Could you check a few things on this model? Use its own coordinates, in mm. A direction names the side the tool comes from. Round coordinates to 2 decimals unless told otherwise and drop trailing zeros. Write each loop counter-clockwise with the first axis right and the second up, starting at its lowest first coordinate (ties: lowest second). Pieces come first, ordered by that corner, then holes. Notation, with made-up numbers: (32, 3) -> (76, 3) arc R21 ccw to (76, 14) -> close; hole circle Ø11 at (-17.5, 71). An arc over 180 degrees is marked (long way). Return JSON: item names as keys, results as strings.
from build123d import *

# Parameters (mm, degrees)
F2_R            = 3.175
F3_DEPTH        = 22.226
F3_COPIES_COUNT = 6


# Not quite as in the source:
# - a pattern or mirror of a feature is missing from the dataset's text; its kind, count and spacing are read off the source's solid


with BuildPart() as f1:
    # F0 (on Front) → F1 (revolve)
    with BuildSketch(Plane.XZ):
        with BuildLine():
            Line((7.8105, 0), (34.1376, 0))
            Line((34.1376, 0), (34.1376, 22.225))
            Line((34.1376, 22.225), (16.6751, 22.225))
            Line((16.6751, 22.225), (16.6751, 14.224))
            ThreePointArc((16.6751, 14.224), (16.2287307345, 13.1463692655), (15.1511, 12.7))
            Line((15.1511, 12.7), (7.8105, 12.7))
            Line((7.8105, 12.7), (7.8105, 0))
        make_face()
    revolve(axis=Axis((0, 0, 6.35), (0, 0, 1)))

    # F2 (on face) → F3 (cut, through all)
    with BuildSketch(Plane.XY.offset(22.225)):
        with Locations((0, 26.2001)):
            Circle(F2_R)
    f3 = extrude(amount=-F3_DEPTH, mode=Mode.SUBTRACT)

    # F3_copies: F3 ×6 about axis
    f3_copies_axis = Axis((0, 0, 0), (0, 0, 1))
    for i in range(1, F3_COPIES_COUNT):
        add(f3.rotate(f3_copies_axis, i * 360 / F3_COPIES_COUNT), mode=Mode.SUBTRACT)


solid = f1.part
1) If I drill on probe 1 along Y at (x, z) = (0, 3); probe 2 along Y at (x, z) = (25.5, 13); probe 3 along X at (y, z) = (12.5, 8.5), over which ranges is the centre line in solid material (lowest first)? Write a range as [from, to].
Return value:
{"probe 1": "[-34.14, -29.38], [-23.03, -7.81], [7.81, 23.03], [29.38, 34.14]", "probe 2": "[-22.7, -14.58], [-11.62, 11.62], [14.58, 22.7]", "probe 3": "[-31.77, -25.81], [-19.57, 19.57], [25.81, 31.77]"}
2) Will these pins go through, and if not, where does the flat tip stop? pin 1 Ø4 at (x, y) = (22.69, 13.1) entering from -Z; pin 2 Ø10 at (x, y) = (0, 26.2) entering from +Z (3 decimals); pin 3 Ø3 at (x, z) = (2.5, 5) entering from -Y; pin 4 Ø8 at (y, z) = (16, 7.5) entering from -X.
Return value:
{"pin 1": "through", "pin 2": "z = 22.225", "pin 3": "y = -34.12", "pin 4": "x = -31.96"}
3) I want a section at A-A, the plane y = 0. Please give me the cut outline in (x, z) (1 decimal).
Return value:
{"outline": "(-34.1, 0) -> (-7.8, 0) -> (-7.8, 12.7) -> (-15.2, 12.7) arc R1.5 cw to (-16.7, 14.2) -> (-16.7, 22.2) -> (-34.1, 22.2) -> close; (7.8, 0) -> (34.1, 0) -> (34.1, 22.2) -> (16.7, 22.2) -> (16.7, 14.2) arc R1.5 cw to (15.2, 12.7) -> (7.8, 12.7) -> close"}
4) I want a section at B-B, the plane x = 0. Please give me the cut outline in (y, z) (1 decimal), and give its area (3 significant figures).
Return value:
{"outline": "(-34.1, 0) -> (-29.4, 0) -> (-29.4, 22.2) -> (-34.1, 22.2) -> close; (-23, 0) -> (-7.8, 0) -> (-7.8, 12.7) -> (-15.2, 12.7) arc R1.5 cw to (-16.7, 14.2) -> (-16.7, 22.2) -> (-23, 22.2) -> close; (7.8, 0) -> (23, 0) -> (23, 22.2) -> (16.7, 22.2) -> (16.7, 14.2) arc R1.5 cw to (15.2, 12.7) -> (7.8, 12.7) -> close; (29.4, 0) -> (34.1, 0) -> (34.1, 22.2) -> (29.4, 22.2) -> close", "area": "720 mm²"}
5) For faces 1 (the face through (-7, 4, 12.7)), 2 (the face through (-8, -15, 22.225)), which set-ups out of +Z, -Z, +X, -X, +Y, -Y let a thin tool reach every point of the face, with its end or its side?
Return value:
{"face 1": "+Z", "face 2": "+Z, +X, -X, +Y, -Y"}
6) I want a section at C-C, the plane z = 18.25. Please give me the cut outline in (x, y) (3 decimals), and give its area (3 significant figures).
Return value:
{"outline": "circle Ø68.275 at (0, 0); hole circle Ø6.35 at (-22.69, -13.1); hole circle Ø6.35 at (-22.69, 13.1); hole circle Ø33.35 at (0, 0); hole circle Ø6.35 at (0, -26.2); hole circle Ø6.35 at (0, 26.2); hole circle Ø6.35 at (22.69, -13.1); hole circle Ø6.35 at (22.69, 13.1)", "area": "2,600 mm²"}
7) I want a section at D-D, the plane z = 2.25. Count the separate pieces of the cut face and the enclosed holes in it, and give its area (3 significant figures).
Return value:
{"separate pieces": "1", "enclosed holes": "7", "area": "3,280 mm²"}
